Could you check a few things on this model? Use its own coordinates, in mm. A direction names the side the tool comes from. Coordinates: 2 decimals unless noted, no trailing zeros. Order: outer loops, then holes, each group sorted by start corner. A loop starts at its lowest first (then second) coordinate and runs counter-clockwise, first axis right, second up. Notation, with made-up numbers: (23.25, 2.25) -> (81.25, 2.25) arc R24 cw to (81.25, 28.25) -> close; hole circle Ø2 at (59.25, -17.75). An arc over 180 degrees is marked (long way). Put each result on its own line as item: value. Start each with the question number.
Q1. Will these pins go through, and if not, where does the flat tip stop? pin 1 (11.5 mm diameter, centred on y = 15.5, z = 17, fed in from -X); pin 2 (4 mm diameter, centred on y = 9, z = 19, fed in from +X); pin 3 (2 mm diameter, centred on x = 15.5, z = 15.5, fed in from +Y).
Q2. If we section it at D-D (x = 9.5): Please give me the cut outline in (y, z) (3 decimals).
Q3. If we section it at B-B (x = 12): Please give me the cut outline in (y, z) (3 decimals), and give its area (3 significant figures).
Q4. For faces 4 (the face through (0, 10, 20)), 5 (the face through (12.91, 10.43, 36.23)), 6 (the face through (13, 2.54, 20)), which set-ups out of +Z, -Z, +X, -X, +Y, -Y let a thin tool reach every point of the face, with its end or its side?
Q5. If we section it at C-C (z = 26.5): Please give me the cut outline in (x, y), and give its area (3 significant figures).
Q6. Please list where these lines run through material, in increasing order: line 1 along Z through (x, y) = (14, 9.25) (3 decimals); line 2 along X through (y, z) = (12.25, 5); line 3 along Y through (x, z) = (10.75, 9.5).
Q7. We'd pull the mould along Z, two halves only. Please class faces 1 (the face through (9, 10, 38.735)), 2 (the face through (5.08, 12, 19)), 3 (the face through (-2.54, 9, 36)): +Z half, -Z half, draft (parallel to the pull), parting line (faces both ways), or undercut.
from build123d import *

# Parameters (mm, degrees)
BOSS_EXTRUDE1_DEPTH = 38.735
SKETCH2_W           = 24.13
SKETCH2_H           = 24.13
SKETCH2_R           = 1.8415
BOSS_EXTRUDE2_DEPTH = 5.08
BOSS_EXTRUDE3_START = -5.08
SKETCH3_W           = 24.13
SKETCH3_H           = 24.13
SKETCH3_R           = 1.8415
BOSS_EXTRUDE3_DEPTH = 5.08
SKETCH4_W           = 38.735
SKETCH4_H           = 5.875923506
BOSS_EXTRUDE5_DEPTH = 21.59
SKETCH5_W           = 28.575
SKETCH5_H           = 2.54
CUT_EXTRUDE1_DEPTH  = 16.51
CHAMFER2_SIZE       = 2.54


with BuildPart() as part:
    # Sketch1 → Boss-Extrude1 (new body)
    with BuildSketch(Plane.XY):
        Polygon((0, 0), (21.59, 0), (21.59, 5.08), (5.08, 5.08), (5.08, 21.59), (0, 21.59), (0, 5.08), align=None)
    extrude(amount=BOSS_EXTRUDE1_DEPTH)

    # Sketch2 → Boss-Extrude2 (add)
    with BuildSketch(Plane.XY.offset(38.735)):
        with Locations((9.525, 9.525)):
            Rectangle(SKETCH2_W, SKETCH2_H)
        with Locations((12.065, 12.065)):
            Circle(SKETCH2_R, mode=Mode.SUBTRACT)
    extrude(amount=-BOSS_EXTRUDE2_DEPTH)

    # Sketch3 → Boss-Extrude3 (add)
    with BuildSketch(Plane(origin=(0, 0, 0), x_dir=(-1, 0, 0), z_dir=(0, 0, -1)).offset(BOSS_EXTRUDE3_START)):
        with Locations((-9.525, 9.525)):
            Rectangle(SKETCH3_W, SKETCH3_H)
        with Locations(Location((-12.065, 12.065, 0), (0, 0, 180))):
            Circle(SKETCH3_R, mode=Mode.SUBTRACT)
    extrude(amount=BOSS_EXTRUDE3_DEPTH)

    # Sketch4 → Boss-Extrude5 (add)
    with BuildSketch(Plane(origin=(21.59, 0, 0), x_dir=(0, 0, -1), z_dir=(1, 0, 0))):
        with Locations((-19.3675, 0.397961753)):
            Rectangle(SKETCH4_W, SKETCH4_H)
    extrude(amount=-BOSS_EXTRUDE5_DEPTH)

    # Sketch5 → Cut-Extrude1 (cut)
    with BuildSketch(Plane(origin=(21.59, 0, 0), x_dir=(0, 0, -1), z_dir=(1, 0, 0))):
        with Locations((-19.3675, 3.81)):
            Rectangle(SKETCH5_W, SKETCH5_H)
    extrude(amount=-CUT_EXTRUDE1_DEPTH, mode=Mode.SUBTRACT)

    # Chamfer2
    chamfer2_edges = [part.edges().sort_by_distance(p)[0] for p in [
        (0, 9.525, 33.655),
        (0, 9.525, 5.08),
    ]]
    chamfer(chamfer2_edges, length=CHAMFER2_SIZE - 0.0001)  # a hair under: the kernel refuses the full size


solid = part.part
The answers:
1. pin 1: x = 0
1. pin 2: x = 5.08
1. pin 3: y = 2.54
2. outline: (-2.54, 0) -> (21.59, 0) -> (21.59, 5.08) -> (2.54, 5.08) -> (2.54, 33.655) -> (21.59, 33.655) -> (21.59, 38.735) -> (-2.54, 38.735) -> close
3. outline: (-2.54, 0) -> (10.225, 0) -> (10.225, 5.08) -> (2.54, 5.08) -> (2.54, 33.655) -> (10.225, 33.655) -> (10.225, 38.735) -> (-2.54, 38.735) -> close; (13.905, 0) -> (21.59, 0) -> (21.59, 5.08) -> (13.905, 5.08) -> close; (13.905, 33.655) -> (21.59, 33.655) -> (21.59, 38.735) -> (13.905, 38.735) -> close
3. area: 353 mm^2
4. face 4: -X, +Y, -Y
4. face 5: +Z, -Z
4. face 6: +X, +Y
5. outline: (0, -2.54) -> (21.59, -2.54) -> (21.59, 2.54) -> (5.08, 2.54) -> (5.08, 21.59) -> (0, 21.59) -> close
5. area: 206 mm^2
6. line 1: 0 to 5.08, 33.655 to 38.735
6. line 2: -2.54 to 10.23, 13.9 to 21.59
6. line 3: -2.54 to 2.54
7. face 1: +Z half
7. face 2: undercut
7. face 3: draft
